Part model, mm, in its own coordinate system. Face numbers are marked on the shaded views. A direction names the side the tool comes from. Give positions to 0.01 mm unless a question says otherwise; leave off trailing zeros. Order: outer loops, then holes, each group sorted by start corner. A loop starts at its lowest first (then second) coordinate and runs counter-clockwise, first axis right, second up. Notation, with made-up numbers: (6, 18.5) - (27, 18.5) arc R20 ccw to (27, 44.5) - close; hole circle Ø9 at (34.5, 66). An arc over 180 degrees is marked (long way). One line per item, written item: value.
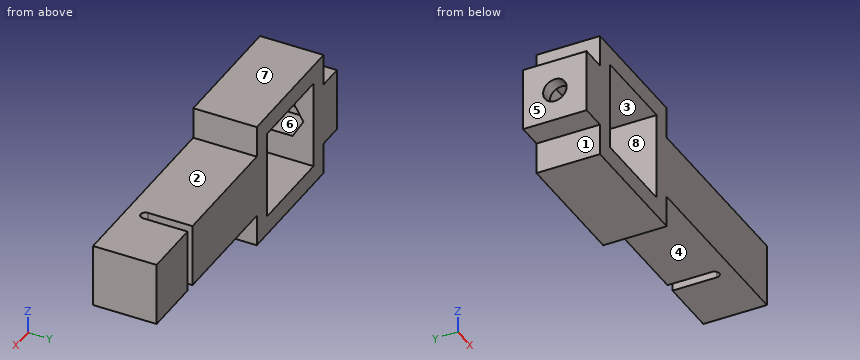
```python
from build123d import *

# Parameters (mm, degrees)
SKETCH1_W           = 14
SKETCH1_H           = 14
BOSS_EXTRUDE1_DEPTH = 10
CUT_EXTRUDE1_REACH  = 37
SKETCH4_R           = 1.85
CUT_EXTRUDE2_DEPTH  = 2
CUT_EXTRUDE3_REACH  = 57.036


with BuildPart() as part:
    # Sketch1 → Boss-Extrude1 (new body)
    with BuildSketch(Plane(origin=(0, 0, 0), x_dir=(1, 0, 0), z_dir=(0, 1, 0))):
        Polygon((0, 0), (30, 0), (30, 10), (0, 10), (0, 15), (-20, 15), (-20, 10), (-24, 10), (-24, 0), (-20, 0), (-20, -5), (0, -5), align=None)
        with Locations((-10, 5)):
            Rectangle(SKETCH1_W, SKETCH1_H, mode=Mode.SUBTRACT)
    extrude(amount=BOSS_EXTRUDE1_DEPTH)

    # Sketch3 → Cut-Extrude1 (cut, up to next)
    with BuildSketch(Plane.XY, mode=Mode.PRIVATE) as cut_extrude1_sk1:
        with BuildLine():
            Line((19.25, 10), (20.75, 10))
            Line((20.75, 10), (20.75, 3))
            ThreePointArc((20.75, 3), (20, 2.25), (19.25, 3))
            Line((19.25, 3), (19.25, 10))
        make_face()
    cut_extrude1_tool1 = extrude(cut_extrude1_sk1.sketch, amount=-CUT_EXTRUDE1_REACH, mode=Mode.PRIVATE) & part.part
    add(cut_extrude1_tool1.solids().sort_by_distance((20, 6.203629, 0))[0], mode=Mode.SUBTRACT)

    # Sketch4 → Cut-Extrude2 (cut)
    with BuildSketch(Plane.ZY.offset(24)):
        with Locations((-5, 5)):
            Circle(SKETCH4_R)
    extrude(amount=-CUT_EXTRUDE2_DEPTH, mode=Mode.SUBTRACT)

    # Sketch5 → Cut-Extrude3 (cut, up to next)
    with BuildSketch(Plane.ZY.offset(22), mode=Mode.PRIVATE) as cut_extrude3_sk1:
        Polygon((-5, 8.4), (-7.944486373, 6.7), (-7.944486373, 3.3), (-5, 1.6), (-2.055513627, 3.3), (-2.055513627, 6.7), align=None)
    cut_extrude3_tool1 = extrude(cut_extrude3_sk1.sketch, amount=-CUT_EXTRUDE3_REACH, mode=Mode.PRIVATE) & part.part
    add(cut_extrude3_tool1.solids().sort_by_distance((-22, 5, -5))[0], mode=Mode.SUBTRACT)


solid = part.part
```
1) Cut at C-C, the plane x = -11.5. Give the cut face in (y, z), then the cut area to 3 significant figures.
Outcome:
outline: (0, -15) - (10, -15) - (10, -12) - (0, -12) - close; (0, 2) - (10, 2) - (10, 5) - (0, 5) - close
area: 60.0 mm^2
2) Which spindle directions (+Z, -Z, +X, -X, +Y, -Y) get a long thin tool onto all of the face, cutting with end or side? Do the marked faces 1, 2, 3 and 4. Say none if no direction does.
Outcome:
face 1: -Z, -X, +Y, -Y
face 2: +Z, +X, +Y, -Y
face 3: +Y, -Y
face 4: -Z, +X, +Y, -Y
3) Cut at B-B, the plane y = 5. Give the cut face in (x, z), then the cut area to 3 significant figures.
Outcome:
outline: (-24, -10) - (-20, -10) - (-20, -15) - (0, -15) - (0, -10) - (19.25, -10) - (19.25, 0) - (0, 0) - (0, 5) - (-20, 5) - (-20, 0) - (-24, 0) - (-24, -3.15) - (-22, -3.15) - (-22, -2.06) - (-17, -2.06) - (-17, 2) - (-3, 2) - (-3, -12) - (-17, -12) - (-17, -7.94) - (-22, -7.94) - (-22, -6.85) - (-24, -6.85) - close; (20.75, -10) - (30, -10) - (30, 0) - (20.75, 0) - close
area: 492 mm^2
4) Cut at A-A, the plane z = -10.5. Give the cut face in (x, y), then the cut area to 3 significant figures.
Outcome:
outline: (-20, 0) - (-17, 0) - (-17, 10) - (-20, 10) - close; (-3, 0) - (0, 0) - (0, 10) - (-3, 10) - close
area: 60.0 mm^2
5) Mould opens along Z. For the marked faces 5, 6, 7 and 8 say: released by +Z, released by -Z, zero draft, split by the parting line, or undercut.
Outcome:
face 5: zero draft
face 6: undercut
face 7: released by +Z
face 8: undercut
6) Drill centre lines: line 1 along X through (y, z) = (8.25, -0.25); line 2 along X through (y, z) = (3.25, -5.5); line 3 along Y through (x, z) = (-22.95, -5). Where is each one in solid material? Low to high. Write a range as from..to.
Outcome:
line 1: x = -24..-17, -3..19.25, 20.75..30
line 2: x = -3..19.25, 20.75..30
line 3: y = 0..3.15, 6.85..10
7) Pin check, flat tips, straight feed: pin 1 (1.5 mm diameter, centred on y = 6, z = -12.5, fed in from +X); pin 2 (4 mm diameter, centred on y = 3.5, z = 2.5, fed in from -X); pin 3 (1.2 mm diameter, centred on x = -22.5, y = 5, fed in from -Z); pin 4 (10 mm diameter, centred on x = 17, z = -3, fed in from -Y). Stop position of each tip, or through.
Outcome:
pin 1: stops at x = 0
pin 2: stops at x = -20
pin 3: stops at z = -10
pin 4: stops at y = 0
8) Cut at D-D, the plane z = 2.5. Give the cut face in (x, y), then the cut area to 3 significant figures.
Outcome:
outline: (-20, 0) - (0, 0) - (0, 10) - (-20, 10) - close
area: 200 mm^2
